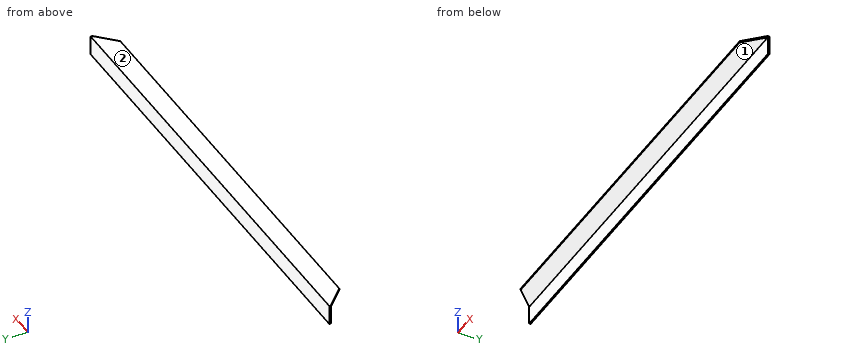
from build123d import *

# Parameters (mm, degrees)
F1_DEPTH = 900
F2_SIZE  = 37
F3_SIZE  = 37


with BuildPart() as f1:
    # F0 (on Right) → F1 (new body)
    with BuildSketch(Plane.YZ):
        Polygon((37, 37), (37, 0), (40, 0), (40, 40), (0, 40), (0, 37), align=None)
    extrude(amount=F1_DEPTH)

    # F2
    f2_edges = [f1.edges().sort_by_distance(p)[0] for p in [
        (900, 0, 38.5),
    ]]
    chamfer(f2_edges, length=F2_SIZE)

    # F3
    f3_edges = [f1.edges().sort_by_distance(p)[0] for p in [
        (0, 0, 38.5),
    ]]
    chamfer(f3_edges, length=F3_SIZE)


solid = f1.part
Input: part model. Units: mm. Frame: model coordinates. Face numbers are marked on the shaded views. A direction names the side the tool comes from. Round coordinates to 2 decimals unless told otherwise and drop trailing zeros. Order: outer loops, then holes, each group sorted by start corner. A loop starts at its lowest first (then second) coordinate and runs counter-clockwise, first axis right, second up. Notation, with made-up numbers: (23.5, 4) - (53.5, 4) arc R26 ccw to (53.5, 36) - close; hole circle Ø5 at (-7.5, -39.75). An arc over 180 degrees is marked (long way). Answer as a JSON object with one key per item and string values. Group by question number.
(1) Pin query (flat end, axial travel): P1, Ø6, axis at y = 12.5, z = 34.5, coming from the +X side; P2, Ø1.5, axis at x = 133, y = 11.5, coming from the -Z side; P3, Ø2, axis at x = 498.5, z = 34.5, coming from the -Y side. Return the tip coordinate at first contact, or that it passes through.
(2) Reachability of the marked faces 1 and 2 from +Z, -Z, +X, -X, +Y, -Y: full face, straight path, thin tool, end or side. Return the list, or none.
(3) Material intervals for probe 1 along Y at (x, z) = (860.5, 6), sorted ascending. Write a range as from..to.
(4) Cut plane C-C (z = 29). Return loops of the section in (x, y).
(5) Cut plane B-B (y = 10). Return loops of the section in (x, z), then the cut area to 3 significant figures.
(6) Cut plane A-A (x = 677). Return loops of the section in (y, z), then the cut area to 3 significant figures.
Here are the results:
{
 "1": {"P1": "stops at x = 877.16", "P2": "stops at z = 37", "P3": "stops at y = 37"},
 "2": {"face 1": "-Z, +X, -X, -Y", "face 2": "+Z, +X, -X, +Y, -Y"},
 "3": {"probe 1": "y = 37..40"},
 "4": {"outline": "(0, 37) - (900, 37) - (900, 40) - (0, 40) - close"},
 "5": {"outline": "(27, 37) - (873, 37) - (873, 40) - (27, 40) - close", "area": "2,540 mm^2"},
 "6": {"outline": "(0, 37) - (37, 37) - (37, 0) - (40, 0) - (40, 40) - (0, 40) - close", "area": "231 mm^2"}
}
